```python
from build123d import *

# Parameters (mm, degrees)
SKETCH1_W           = 200
SKETCH1_H           = 30
SKETCH1_W_2         = 40
SKETCH1_H_2         = 13
SKETCH1_W_3         = 4
SKETCH1_H_3         = 10
BOSS_EXTRUDE1_DEPTH = 4


with BuildPart() as part:
    # Sketch1 → Boss-Extrude1 (new body)
    # profile 1 of 5: a face of its own
    with BuildSketch(Plane(origin=(0, 0, 0), x_dir=(1, 0, 0), z_dir=(0, 1, 0))):
        with Locations((100, 15)):
            Rectangle(SKETCH1_W, SKETCH1_H)
        with Locations((45, 15)):
            Rectangle(SKETCH1_W_2, SKETCH1_H_2, mode=Mode.SUBTRACT)
    # profile 2 of 5: a face of its own
    with BuildSketch(Plane(origin=(0, 0, 0), x_dir=(1, 0, 0), z_dir=(0, 1, 0))):
        with Locations((-2, 5)):
            Rectangle(SKETCH1_W_3, SKETCH1_H_3)
    # profile 3 of 5: a face of its own
    with BuildSketch(Plane(origin=(0, 0, 0), x_dir=(1, 0, 0), z_dir=(0, 1, 0))):
        with Locations((-2, 25)):
            Rectangle(SKETCH1_W_3, SKETCH1_H_3)
    # profile 4 of 5: a face of its own
    with BuildSketch(Plane(origin=(0, 0, 0), x_dir=(1, 0, 0), z_dir=(0, 1, 0))):
        with Locations((202, 25)):
            Rectangle(SKETCH1_W_3, SKETCH1_H_3)
    # profile 5 of 5: a face of its own
    with BuildSketch(Plane(origin=(0, 0, 0), x_dir=(1, 0, 0), z_dir=(0, 1, 0))):
        with Locations((202, 5)):
            Rectangle(SKETCH1_W_3, SKETCH1_H_3)
    extrude(amount=BOSS_EXTRUDE1_DEPTH)


solid = part.part
```
Model file for the job. Use its own axes, mm. A direction names the side the tool comes from. Coordinates: 2 decimals unless noted, no trailing zeros. Loops run counter-clockwise (first coordinate to the right, second up) from the corner with the lowest first, then second, coordinate; pieces in that order, holes last. Notation, with made-up numbers: (13, -40) - (67, -40) arc R17 ccw to (67, -21) - close; hole circle Ø3 at (11.5, 78). An arc over 180 degrees is marked (long way). Write item = value, one per line. Start each with the question number.
Item 1: Saw through at B-B, the plane y = 1.3. List the corners of the cut face in (x, z), then the cut area to 3 significant figures.
Item 2: Saw through at A-A, the plane z = -12.25. List the corners of the cut face in (x, y).
Item 3: Pull direction Z, two halves, no side cores. Call faces 1 (the face through (200, 2, -15)), 2 (the face through (204, 2, -5)), 3 (the face through (99, 2, 0)): +Z half, -Z half, draft (parallel to the pull), parting line (faces both ways), or undercut.
Item 4: Drop flat-ended pins along their axis: pin 1 Ø1.5 at (y, z) = (1, -19) entering from +X; pin 2 Ø2 at (y, z) = (1, -15.5) entering from -X. Give the stop position or say it passes through.
Item 5: 3-axis set-ups, long thin cutter, end or side, ignore diameter. For faces 4 (the face through (-2, 2, -20)), 5 (the face through (65, 2, -15)), 6 (the face through (202, 2, -20)): which of +Z, -Z, +X, -X, +Y, -Y reach the whole face in a straight line?
Item 6: Wall check: probe 1 along X at (y, z) = (2.1, -16.5); probe 2 along Z at (x, y) = (46.5, 2.5). Give the ranges that are in metal, low to high. Write a range as [from, to].
Answers:
q1.outline = (-4, -30) - (204, -30) - (204, -20) - (200, -20) - (200, -10) - (204, -10) - (204, 0) - (-4, 0) - (-4, -10) - (0, -10) - (0, -20) - (-4, -20) - close; hole (25, -21.5) - (65, -21.5) - (65, -8.5) - (25, -8.5) - close
q1.area = 5,640 mm2
q2.outline = (0, 0) - (25, 0) - (25, 4) - (0, 4) - close; (65, 0) - (200, 0) - (200, 4) - (65, 4) - close
q3.face_1 = undercut
q3.face_2 = draft
q3.face_3 = +Z half
q4.pin_1 = 200
q4.pin_2 = 0
q5.face_4 = -X, +Y, -Y
q5.face_5 = +Y, -Y
q5.face_6 = +X, +Y, -Y
q6.probe_1 = [0, 25], [65, 200]
q6.probe_2 = [-30, -21.5], [-8.5, 0]
